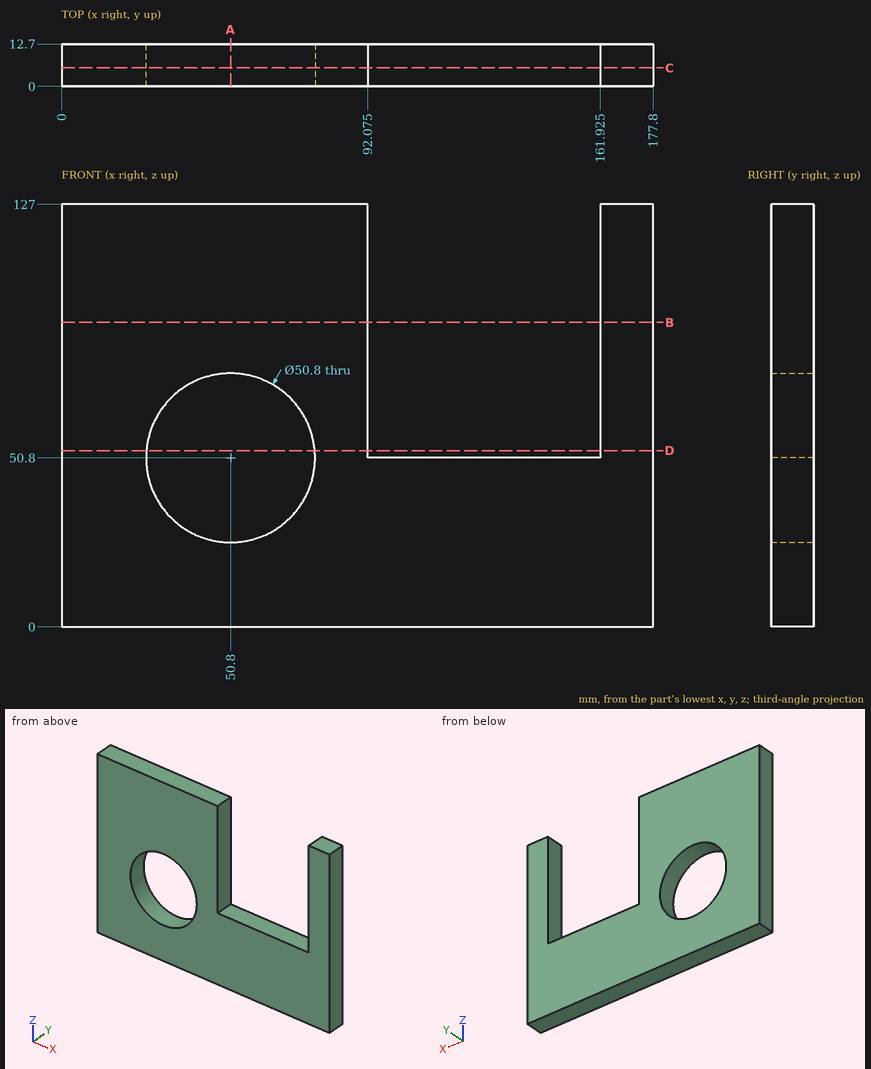
Drawing for the job (mm, zero at the part's lowest x, y, z). Give positions to 0.01 mm unless a question says otherwise; leave off trailing zeros. Loops run counter-clockwise (first coordinate to the right, second up) from the corner with the lowest first, then second, coordinate; pieces in that order, holes last. Notation, with made-up numbers: M 42.5,65 L 100.5,65 A13 ccw 100.5,83 Z; hole C 26,1.5 d10. An arc over 180 degrees is marked long. One line per question, with ' | ' between items. Start each with the question number.
1. Saw through at D-D on z = 53. Give the cut face in (x, y) (3 decimals).
2. Probe L1, parallel to X at y = 3.5, z = 101 (3 decimals); L2, parallel to Z at x = 50.8, y = 3.25; L3, parallel to X at y = 12, z = 70 (3 decimals). List the from-to ranges inside material, lowest first. Write a range as from..to.
3. Flat gauge pin, fed straight in: pin 1 (1.5 mm diameter, centred on x = 95.5, y = 6.5, fed in from +Z). Where does the tip first touch, or does it go through?
4. Saw through at A-A on x = 50.8. Give the cut face in (y, z), plus the area to 3 significant figures.
5. Saw through at B-B on z = 91.5. Give the cut face in (x, y) (3 decimals), plus the area to 3 significant figures.
6. Saw through at C-C on y = 5.5. Give the cut face in (x, z) (3 decimals).
Result sheet:
1) outline: M 0,0 L 25.495,0 L 25.495,12.7 L 0,12.7 Z; M 76.105,0 L 92.075,0 L 92.075,12.7 L 76.105,12.7 Z; M 161.925,0 L 177.8,0 L 177.8,12.7 L 161.925,12.7 Z
2) L1: x = 0..92.075, 161.925..177.8 | L2: z = 0..25.4, 76.2..127 | L3: x = 0..34.171, 67.429..92.075, 161.925..177.8
3) pin 1: stops at z = 50.8
4) outline: M 0,0 L 12.7,0 L 12.7,25.4 L 0,25.4 Z; M 0,76.2 L 12.7,76.2 L 12.7,127 L 0,127 Z | area: 968 mm^2
5) outline: M 0,0 L 92.075,0 L 92.075,12.7 L 0,12.7 Z; M 161.925,0 L 177.8,0 L 177.8,12.7 L 161.925,12.7 Z | area: 1,370 mm^2
6) outline: M 0,0 L 177.8,0 L 177.8,127 L 161.925,127 L 161.925,50.8 L 92.075,50.8 L 92.075,127 L 0,127 Z; hole C 50.8,50.8 d50.8
